```python
from build123d import *

# Parameters (mm, degrees)
F0_W     = 116.7713552713
F0_H     = 81.8841084838
F1_DEPTH = 63.5
F2_W     = 101.201839745
F2_H     = 68.6211884022
F3_DEPTH = 76.2
F4_W     = 37.7704855055
F4_H     = 26.3061614931
F5_DEPTH = 101.6
F6_R     = 10.7156229068
F7_DEPTH = 101.6
F8_R     = 10.8160051842
F9_DEPTH = 101.6


with BuildPart() as f1:
    # F0 (on Top) → F1 (new body)
    with BuildSketch(Plane.XY):
        Rectangle(F0_W, F0_H)
    extrude(amount=F1_DEPTH)

    # F2 (on face) → F3 (cut)
    with BuildSketch(Plane.XY.offset(63.5)):
        Rectangle(F2_W, F2_H)
    extrude(amount=-F3_DEPTH, mode=Mode.SUBTRACT)

    # F4 (on face) → F5 (cut)
    with BuildSketch(Plane.XZ.offset(40.9420542419)):
        with Locations((3.4598903731, 50.3469192535)):
            Rectangle(F4_W, F4_H)
    extrude(amount=-F5_DEPTH, mode=Mode.SUBTRACT)

    # F6 (on face) → F7 (cut)
    with BuildSketch(Plane(origin=(-58.3856776357, 0, 0), x_dir=(0, -1, 0), z_dir=(-1, 0, 0))):
        with Locations((0, 35.4638919234)):
            Circle(F6_R)
    extrude(amount=-F7_DEPTH, mode=Mode.SUBTRACT)

    # F8 (on face) → F9 (cut)
    with BuildSketch(Plane.YZ.offset(58.3856776357)):
        with Locations((0, 36.3288670778)):
            Circle(F8_R)
    extrude(amount=-F9_DEPTH, mode=Mode.SUBTRACT)


solid = f1.part
```
Here's how the part is built. I have some questions about the finished solid (model axes, mm). A direction names the side the tool comes from. Round coordinates to 2 decimals unless told otherwise and drop trailing zeros. Order: outer loops, then holes, each group sorted by start corner. A loop starts at its lowest first (then second) coordinate and runs counter-clockwise, first axis right, second up. Notation, with made-up numbers: M -12.75,-9.75 L -7.75,-9.75 A32 cw -7.75,25.25 Z; hole C -35.5,87.5 d7. An arc over 180 degrees is marked long. Answer in a Markdown table with one row per item.
Item 1: For faces 4 (the face through (54.55, -2.34, 25.77)), 5 (the face through (3, -38, 37.194)), 6 (the face through (-54.55, 1.39, 46.09)), 7 (the face through (-50.601, -8, 25)), 8 (the face through (-1, -36, 0)), which set-ups out of +Z, -Z, +X, -X, +Y, -Y let a thin tool reach every point of the face, with its end or its side?
A:
| item | result |
|---|---|
| face 4 | +X |
| face 5 | +Z, +Y, -Y |
| face 6 | -X |
| face 7 | +Z, -Z |
| face 8 | -Z, +X, -X, +Y, -Y |
Item 2: Imagine slicing it at A-A, the plane x = 25. Write out the boundary of the cut face in (y, z), and give its area (3 significant figures).
A:
| item | result |
|---|---|
| outline | M -40.94,0 L -34.31,0 L -34.31,63.5 L -40.94,63.5 Z; M 34.31,0 L 40.94,0 L 40.94,63.5 L 34.31,63.5 Z |
| area | 842 mm2 |
Item 3: I'm going to push a flat-ended pin straight in: pin 1 (7.5 mm diameter, centred on x = 12, y = 37.5, fed in from +Z). Where does the tip first touch, or does it pass through?
A:
| item | result |
|---|---|
| pin 1 | stops at z = 37.19 |
Item 4: Imagine slicing it at D-D, the plane y = 0. Write out the boundary of the cut face in (x, z), and give its area (3 significant figures).
A:
| item | result |
|---|---|
| outline | M -58.39,0 L -50.6,0 L -50.6,24.75 L -58.39,24.75 Z; M -58.39,46.18 L -50.6,46.18 L -50.6,63.5 L -58.39,63.5 Z; M 50.6,0 L 58.39,0 L 58.39,25.51 L 50.6,25.51 Z; M 50.6,47.14 L 58.39,47.14 L 58.39,63.5 L 50.6,63.5 Z |
| area | 653 mm2 |
Item 5: Imagine slicing it at C-C, the plane y = -23.5. Write out the boundary of the cut face in (x, z).
A:
| item | result |
|---|---|
| outline | M -58.39,0 L -50.6,0 L -50.6,63.5 L -58.39,63.5 Z; M 50.6,0 L 58.39,0 L 58.39,63.5 L 50.6,63.5 Z |
Item 6: If I drill on L1, parallel to Z at x = 53.25, y = 0; L2, parallel to X at y = -20, z = 26.5; L3, parallel to Y at x = -34.5, z = 54.5, over which ranges is the centre line in solid material (lowest first)? Write a range as from..to.
A:
| item | result |
|---|---|
| L1 | z = 0..25.51, 47.14..63.5 |
| L2 | x = -58.39..-50.6, 50.6..58.39 |
| L3 | y = -40.94..-34.31, 34.31..40.94 |
Item 7: Imagine slicing it at B-B, the plane z = 51.5. Write out the boundary of the cut face in (x, y).
A:
| item | result |
|---|---|
| outline | M -58.39,-40.94 L -15.43,-40.94 L -15.43,-34.31 L -50.6,-34.31 L -50.6,34.31 L -15.43,34.31 L -15.43,40.94 L -58.39,40.94 Z; M 22.35,-40.94 L 58.39,-40.94 L 58.39,40.94 L 22.35,40.94 L 22.35,34.31 L 50.6,34.31 L 50.6,-34.31 L 22.35,-34.31 Z |
Item 8: Thinking about a two-plate mould opening in Y: for faces 1 (the face through (50.601, 0, 25)), 2 (the face through (-1, -40.942, 31)), 3 (the face through (-52, 1, 63.5)), which applies, +Y half, -Y half, draft (parallel to the pull), parting line (faces both ways), or undercut?
A:
| item | result |
|---|---|
| face 1 | undercut |
| face 2 | -Y half |
| face 3 | draft |
